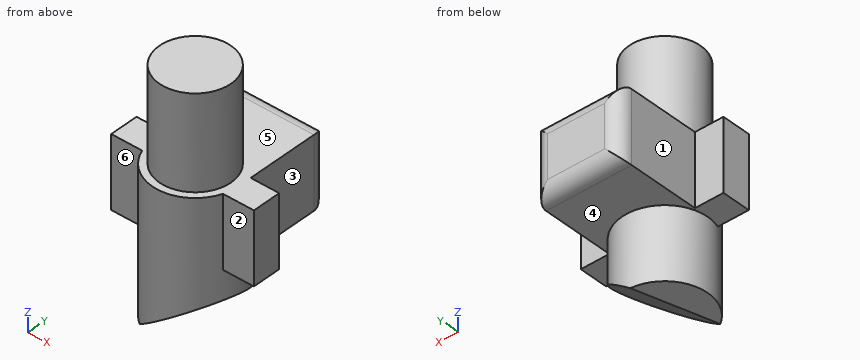
Autodesk Inventor part; units mm, degrees
ref_plane "作業平面2" through (0, 0, 0) normal (0, 1, 0) x (-1, 0, 0)
ref_plane "作業平面3" through (-3, 0, -10) normal (-1, 0, 0) x (0, -1, 0)
ref_plane "作業平面6" through (0.7765, 2.8978, -10) normal (-0.2588, -0.9659, 0) x (0.9659, -0.2588, 0)
sketch "スケッチ1" plane through (0, 0, 0) normal (0, 0, 1) x (1, 0, 0)
  point P0 (0, 0)
sketch "スケッチ2" plane through (0, 0, 0) normal (0, 0, 1) x (1, 0, 0)
  circle A0 centre (0, 0) radius 2.5
  dimension "d0" = 5
extrude "押し出し1" add sketch "スケッチ2" along normal blind 6.5
sketch "スケッチ3" plane through (0, 0, 0) normal (0, 0, -1) x (-1, 0, 0)
  circle A0 centre (0, 0) radius 3
  dimension "d3" = 6
extrude "押し出し2" add sketch "スケッチ3" along normal blind 10
sketch "スケッチ4" plane through (0, 0, 0) normal (0, 0, 1) x (1, 0, 0)
  circle A0 centre (0, 0) radius 3
  point P0 (0, 3)
ref_plane "作業平面2" through (0, 0, 0) normal (0, 1, 0) x (-1, 0, 0)
ref_plane "作業平面1" through (0, 3, 0) normal (0, 1, 0) x (-1, 0, 0)
sketch "スケッチ5" plane through (0, 0, 0) normal (0, 1, 0) x (-1, 0, 0)
  line L0 (5, -5) -> (-5, -5)
  line L1 (-5, -5) -> (-5, 0)
  line L2 (-5, 0) -> (5, 0)
  line L3 (5, 0) -> (5, -5)
  point P0 (0, 0)
  dimension "d7" = 10
  dimension "d8" = 5
  dimension "d9" = 5
extrude "押し出し3" add sketch "スケッチ5" along normal mid plane 2
sketch "スケッチ6" plane through (0, 0, 0) normal (0, 1, 0) x (-1, 0, 0)
  line L0 (5, -5) -> (2.8284, -5)
  line L1 (-2.8284, 0) -> (-5, 0)
  line L2 (3, -5) -> (-3.9142, -5)
  line L3 (-3.9142, -5) -> (-3.9142, 0)
  line L4 (-3.9142, 0) -> (3, 0)
  line L5 (3, 0) -> (3, -5)
  line L6 (3.5037, -5) -> (-3, -5)
  line L7 (-3, -5) -> (-3, 0)
  line L8 (-3, 0) -> (3.5037, 0)
  line L9 (3.5037, 0) -> (3.5037, -5)
  point P0 (0, 0)
  dimension "d12" = 6
  dimension "d13" = 3
extrude "押し出し4" add sketch "スケッチ6" along normal blind 7 contours L0 L2 L7 L1 L4 L5
fillet "フィレット1" radius 1 4 edges at (0, 7, 0) (-3, 7, -2.5) (0, 7, -5) (3, 7, -2.5)
sketch "スケッチ7" plane through (0, 0, -10) normal (0, 0, -1) x (-1, 0, 0)
  arc A0 (2.8284, -1) -> (-2.8284, -1) centre (0, 0) ccw
  point P0 (3, 0)
ref_plane "作業平面3" through (-3, 0, -10) normal (-1, 0, 0) x (0, -1, 0)
sketch "スケッチ12" plane through (0, 0, -10) normal (0, 0, -1) x (-1, 0, 0)
  circle A0 centre (0, 0) radius 3 construction
  arc A1 (2.8284, -1) -> (-2.8284, -1) centre (0, 0) ccw construction
  line L0 (-0.7765, 2.8978) -> (0.7765, -2.8978) construction
  circle A2 centre (0, 0) radius 3 construction
  line L1 (3, 0) -> (-3, 0) construction
  dimension "d22" = 105
ref_plane "作業平面6" through (0.7765, 2.8978, -10) normal (-0.2588, -0.9659, 0) x (0.9659, -0.2588, 0)
sketch "スケッチ13" plane through (0.7765, 2.8978, -10) normal (-0.2588, -0.9659, 0) x (0.9659, -0.2588, 0)
  line L0 (-3, 0) -> (3, 0)
  line L1 (3, 0) -> (3, 3)
  line L2 (3, 5) -> (3, 0)
  line L3 (3, 0) -> (-1, 0)
  line L4 (-1, 0) -> (3, 3)
  point P0 (0, 10)
  dimension "d23" = 3
  dimension "d24" = 4
extrude "押し出し6" cut sketch "スケッチ13" along normal through all
properties part number "スライド"
Input: part model. Units: mm. Frame: model coordinates. Face numbers are marked on the shaded views. A direction names the side the tool comes from. Coordinates: 2 decimals unless noted, no trailing zeros. Loops run counter-clockwise (first coordinate to the right, second up) from the corner with the lowest first, then second, coordinate; pieces in that order, holes last. Notation, with made-up numbers: (-31.5, 23.5) - (23.5, 23.5) arc R20 ccw to (23.5, 39.5) - close; hole circle Ø9 at (3.5, -0.5). An arc over 180 degrees is marked (long way). Answer in a Markdown table with one row per item.
(1) Mould query, pull axis Z, two halves, no side actions, for the marked faces 4, 5 and 6. Classes: pulls with the +Z half, pulls with the -Z half, needs draft (parallel to the pull), parting line crosses it, or undercut.
Model answer:
| item | result |
|---|---|
| face 4 | pulls with the -Z half |
| face 5 | pulls with the +Z half |
| face 6 | needs draft |
(2) Cut plane B-B on x = -2.25. Output: boundary loops of the cut face in (y, z).
Model answer:
| item | result |
|---|---|
| outline | (-1.98, -10) - (1.98, -10) - (1.98, -5) - (6, -5) arc R1 ccw to (6.97, -4.25) - (6.97, -0.75) arc R1 ccw to (6, 0) - (1.09, 0) - (1.09, 6.5) - (-1.09, 6.5) - (-1.09, 0) - (-1.98, 0) - close |
(3) Cut plane C-C on z = -8.5. Output: boundary loops of the cut face in (x, y).
Model answer:
| item | result |
|---|---|
| outline | (0.23, -2.99) - (1.7, 2.47) arc R3 ccw (long way) to start |
(4) Set-up query: the marked faces 1, 2 and 3. Return all of +Z, -Z, +X, -X, +Y, -Y with unobstructed straight access to the full face (end or side cutting, diameter ignored); none if empty.
Model answer:
| item | result |
|---|---|
| face 1 | +Z, -Z, -X, +Y |
| face 2 | +Z, -Z, +X, -Y |
| face 3 | +Z, -Z, +X, +Y |
(5) Cut plane D-D on y = -1.5. Output: boundary loops of the cut face in (x, z).
Model answer:
| item | result |
|---|---|
| outline | (-2.6, -10) - (-1.44, -10) - (2.6, -7.08) - (2.6, 0) - (2, 0) - (2, 6.5) - (-2, 6.5) - (-2, 0) - (-2.6, 0) - close |
(6) Material intervals for L1, parallel to Z at x = -1.5, y = 3.5; L2, parallel to Y at x = 1.5, z = 2.75; L3, parallel to X at y = 4, z = -0.25, sorted ascending. Write a range as from..to.
Model answer:
| item | result |
|---|---|
| L1 | z = -5..0 |
| L2 | y = -2..2 |
| L3 | x = -3..3 |
(7) Pin query (flat end, axial travel): P1, Ø0.6, axis at x = 4.5, z = -2.5, coming from the +Y side; P2, Ø1.5, axis at y = 0.5, z = -6.5, coming from the -X side; P3, Ø1.5, axis at x = -2, z = -6, coming from the +Y side. Return the tip coordinate at first contact, or that it passes through.
Model answer:
| item | result |
|---|---|
| P1 | stops at y = 1 |
| P2 | stops at x = -3 |
| P3 | stops at y = 2.73 |
(8) Cut plane A-A on y = 2. Output: boundary loops of the cut face in (x, z).
Model answer:
| item | result |
|---|---|
| outline | (-3, -5) - (-2.24, -5) - (-2.24, -10) - (-0.5, -10) - (2.24, -8.02) - (2.24, -5) - (3, -5) - (3, 0) - (1.5, 0) - (1.5, 6.5) - (-1.5, 6.5) - (-1.5, 0) - (-3, 0) - close |
